Geometry check sheet. Reference: drawing and pictorial views, mm from the part's lowest x, y, z. A direction names the side the tool comes from. Round coordinates to 2 decimals unless told otherwise and drop trailing zeros. Write each loop counter-clockwise with the first axis right and the second up, starting at its lowest first coordinate (ties: lowest second). Pieces come first, ordered by that corner, then holes. Notation, with made-up numbers: (9, -27.75) - (42, -27.75) arc R7 cw to (42, -21.75) - close; hole circle Ø3 at (-6, -35). An arc over 180 degrees is marked (long way). Use one line per item in the form item = value. Start each with the question number.
1) Gauge pin test, flat ends, axial feed: P1, Ø6, axis at x = 21, z = 41, coming from the +Y side; P2, Ø8, axis at y = 5.5, z = 25.5, coming from the +X side; P3, Ø15, axis at x = 24.5, z = 39.5, coming from the -Y side. Record the tip position at first contact, or that the pin passes through.
2) Scan lines: probe 1 along X at (y, z) = (30, 40.5); probe 2 along X at (y, z) = (9.5, 25); probe 3 along Y at (x, z) = (77.5, 51.5). Record each from-to range of solid material in increasing order.
3) Section check B-B (y = 4.5). Record the boundary of the cut face in (x, z), then the cut area to 3 significant figures.
4) Set-up check for the marked faces 4, 5, 6, 7 and 8: record each of +Z, -Z, +X, -X, +Y, -Y from which the full face is reachable in a straight line by a thin tool's end or side.
5) Section check A-A (x = 103.5). Record the boundary of the cut face in (y, z).
6) Section check C-C (z = 48.5). Record the boundary of the cut face in (x, y).
7) Section check D-D (y = 28.5). Record the boundary of the cut face in (x, z), then the cut area to 3 significant figures.
8) Draft check along Z on the marked faces 1, 2 and 3. Enter one of: +Z half, -Z half, draft (parallel to the pull), parting line (faces both ways), or undercut.
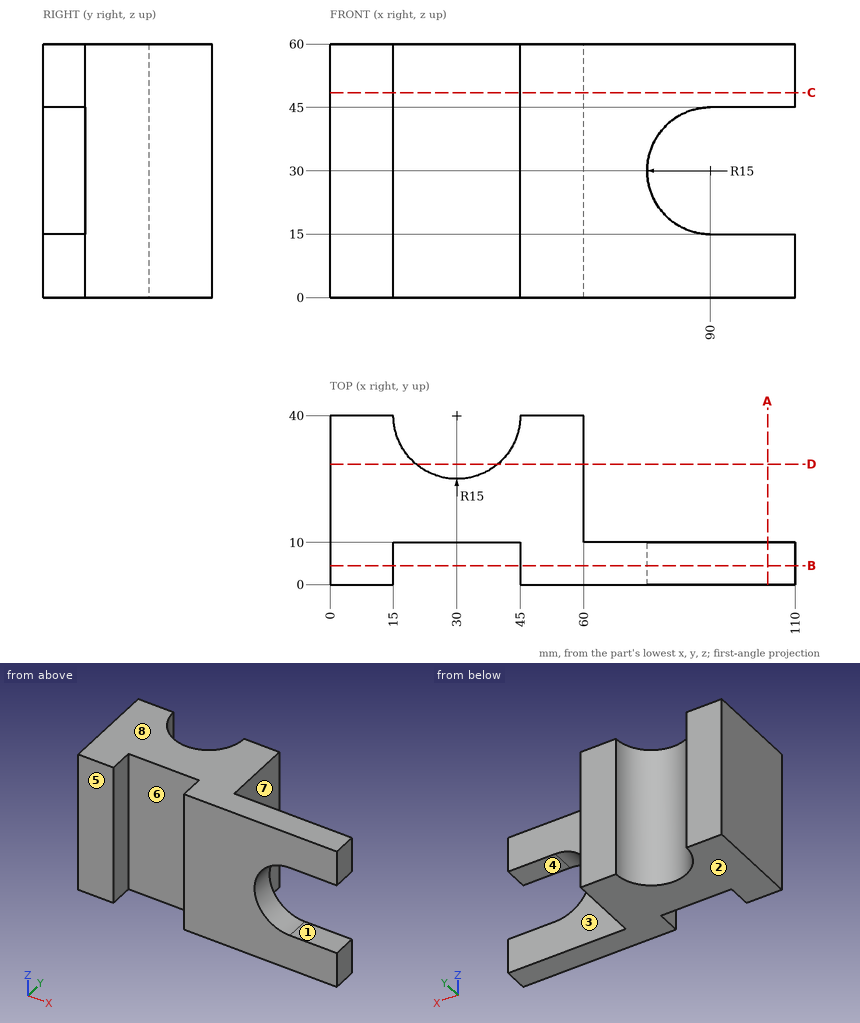
Results are:
q1.P1 = 31
q1.P2 = 77.64
q1.P3 = 10
q2.probe_1 = 0 to 18.82, 41.18 to 60
q2.probe_2 = 0 to 15, 45 to 75.86
q2.probe_3 = 0 to 10
q3.outline = (0, 0) - (15, 0) - (15, 60) - (0, 60) - close; (45, 0) - (110, 0) - (110, 15) - (90, 15) arc R15 cw to (90, 45) - (110, 45) - (110, 60) - (45, 60) - close
q3.area = 3,850 mm²
q4.face_4 = +X, +Y, -Y
q4.face_5 = +Z, -Z, +X, -X, -Y
q4.face_6 = +Z, -Z, -Y
q4.face_7 = +Z, -Z, +X, +Y
q4.face_8 = +Z, +X, -X, +Y, -Y
q5.outline = (0, 0) - (10, 0) - (10, 15) - (0, 15) - close; (0, 45) - (10, 45) - (10, 60) - (0, 60) - close
q6.outline = (0, 0) - (15, 0) - (15, 10) - (45, 10) - (45, 0) - (110, 0) - (110, 10) - (60, 10) - (60, 40) - (45, 40) arc R15 cw to (15, 40) - (0, 40) - close
q7.outline = (0, 0) - (20.37, 0) - (20.37, 60) - (0, 60) - close; (39.63, 0) - (60, 0) - (60, 60) - (39.63, 60) - close
q7.area = 2,440 mm²
q8.face_1 = undercut
q8.face_2 = -Z half
q8.face_3 = draft
